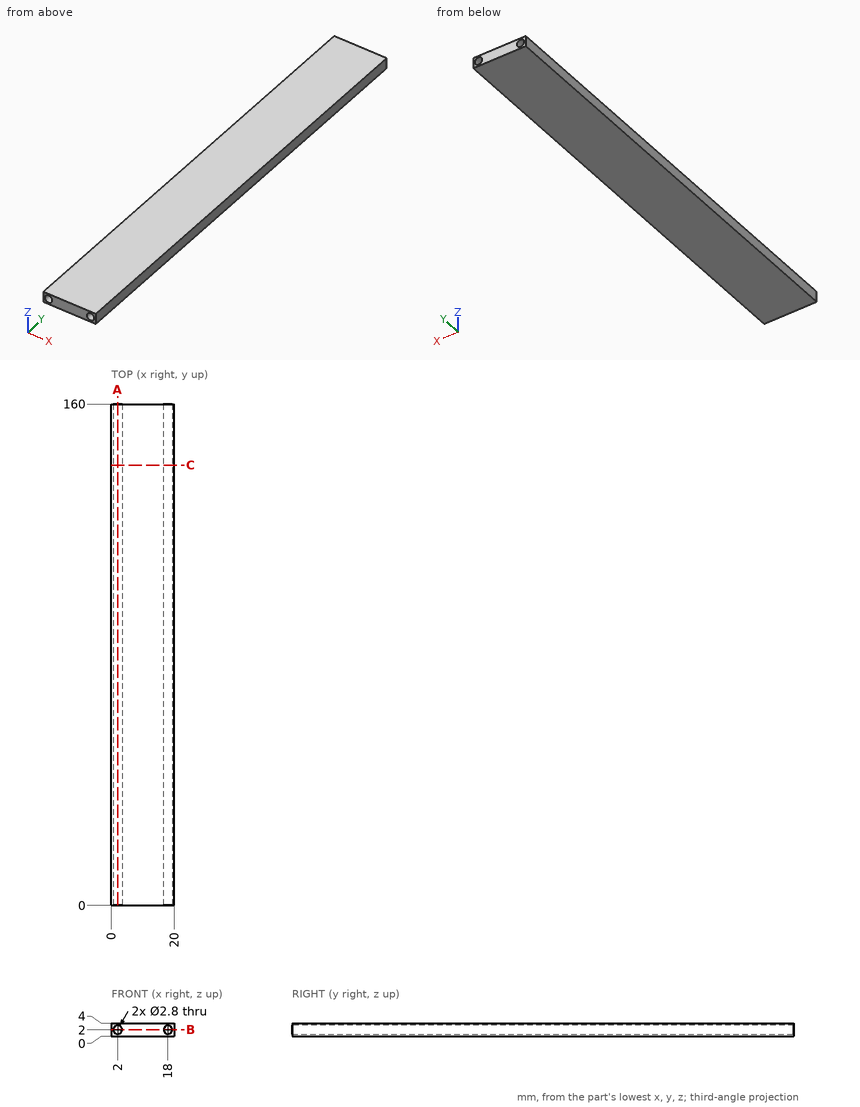
Source: three-view drawing plus pictorial views. Frame: mm from the lowest corner of the part. Coordinates: 2 decimals unless noted, no trailing zeros. Write each loop counter-clockwise with the first axis right and the second up, starting at its lowest first coordinate (ties: lowest second). Pieces come first, ordered by that corner, then holes. Notation, with made-up numbers: (45.25, 70) -> (77.25, 70) arc R10 cw to (77.25, 85) -> close; hole circle Ø3 at (-30, -7.5). An arc over 180 degrees is marked (long way). Answer as a JSON object with one key per item and string values.
1. Section B-B on z = 2. Return the cut outline in (x, y).
Result set:
{"outline": "(0, 0) -> (0.6, 0) -> (0.6, 160) -> (0, 160) -> close; (3.4, 0) -> (16.6, 0) -> (16.6, 160) -> (3.4, 160) -> close; (19.4, 0) -> (20, 0) -> (20, 160) -> (19.4, 160) -> close"}
2. First-contact query: P1, Ø10, axis at x = 17, y = 27, coming from the -Z side. Flat tip, straight axial feed; report the tip coordinate or a pass-through.
Result set:
{"P1": "stops at z = 0"}
3. Material intervals for line 1 (X direction, y = 26, z = 2); line 2 (X direction, y = 38, z = 0.8); line 3 (Z direction, x = 17, y = 63.5), sorted ascending. Write a range as from..to.
Result set:
{"line 1": "x = 0..0.6, 3.4..16.6, 19.4..20", "line 2": "x = 0..1.28, 2.72..17.28, 18.72..20", "line 3": "z = 0..1.02, 2.98..4"}
4. Section C-C on y = 140.5. Return the cut outline in (x, z), then the cut area to 3 significant figures.
Result set:
{"outline": "(0, 0) -> (20, 0) -> (20, 4) -> (0, 4) -> close; hole circle Ø2.8 at (2, 2); hole circle Ø2.8 at (18, 2)", "area": "67.7 mm2"}
5. Section A-A on x = 2. Return the cut outline in (y, z).
Result set:
{"outline": "(0, 0) -> (160, 0) -> (160, 0.6) -> (0, 0.6) -> close; (0, 3.4) -> (160, 3.4) -> (160, 4) -> (0, 4) -> close"}
